```python
from build123d import *

# Parameters (mm, degrees)
SKETCH_4_W           = 84.916455131
SKETCH_4_H           = 80
SKETCH_4_R           = 3
EXTRUDE_1_DEPTH      = 5
EXTRUDE_2_DEPTH      = 3
EXTRUDE_2_DEPTH_BACK = 5
SKETCH_5_R           = 3


with BuildPart() as part:
    # 草图4 → 凸台-拉伸1 (new body)
    with BuildSketch(Plane(origin=(0, 0, 0), x_dir=(1, 0, 0), z_dir=(0, 1, 0))):
        with Locations((-1.967483917, -58.11712094)):
            Rectangle(SKETCH_4_W, SKETCH_4_H)
        with Locations(Location((-36.585071707, -25.636349073, 0), (0, 0, 270))):
            Circle(SKETCH_4_R, mode=Mode.SUBTRACT)
        with Locations(Location((32.601613083, -25.636349073, 0), (0, 0, 270))):
            Circle(SKETCH_4_R, mode=Mode.SUBTRACT)
        with Locations(Location((-36.585071707, -90.861964123, 0), (0, 0, 270))):
            Circle(SKETCH_4_R, mode=Mode.SUBTRACT)
        with Locations(Location((32.601613083, -90.861964123, 0), (0, 0, 270))):
            Circle(SKETCH_4_R, mode=Mode.SUBTRACT)
    extrude(amount=EXTRUDE_1_DEPTH)

    # 草图5 → 凸台-拉伸2 (add, two sides: drawn at the far end of the back side and taken through both)
    with BuildSketch(Plane(origin=(0, 5, 0), x_dir=(1, 0, 0), z_dir=(0, 1, 0)).offset(-EXTRUDE_2_DEPTH_BACK)):
        with Locations(Location((-36.585071707, -25.636349073, 0), (0, 0, 270))):
            Circle(SKETCH_5_R)
        with Locations(Location((32.601613083, -25.636349073, 0), (0, 0, 270))):
            Circle(SKETCH_5_R)
        with Locations(Location((-36.585071707, -90.861964123, 0), (0, 0, 270))):
            Circle(SKETCH_5_R)
        with Locations(Location((32.601613083, -90.861964123, 0), (0, 0, 270))):
            Circle(SKETCH_5_R)
    extrude(amount=EXTRUDE_2_DEPTH + EXTRUDE_2_DEPTH_BACK)


solid = part.part
```
The listing builds one solid part. Answer for the finished solid, in the listing's coordinates (mm). A direction names the side the tool comes from. Coordinates: 2 decimals unless noted, no trailing zeros. Loops run counter-clockwise (first coordinate to the right, second up) from the corner with the lowest first, then second, coordinate; pieces in that order, holes last. Notation, with made-up numbers: (54.25, -22) -> (101.25, -22) arc R14 cw to (101.25, -12) -> close; hole circle Ø6 at (5, 36.25). An arc over 180 degrees is marked (long way). Use one line per item in the form item = value. Start each with the question number.
Item 1: The part is cut by section A-A on z = 80. Determine the outline of the cut face in (x, y).
Item 2: The part is cut by section B-B on y = 7. Determine the outline of the cut face in (x, z).
Item 3: A tool of negligible diameter and unlimited length cuts with its end or side. For faces 5 (the face through (-37, 8, 26)), 6 (the face through (34.63, 6.48, 88.65)), from which of +Z, -Z, +X, -X, +Y, -Y can it reach the whole face along a straight path? Write none if from no direction.
Item 4: The mould has two halves that part along Z. Classify faces 1 (the face through (-3, 2, 18.117)), 2 (the face through (-34.055, 6.479, 27.249)), 3 (the face through (35.13, 6.48, 27.25)), 4 (the face through (33, 8, 26)): released by +Z, released by -Z, zero draft, split by the parting line, or undercut.
Item 5: Consider L1, parallel to Y at x = -10, z = 35; L2, parallel to X at y = 5.75, z = 92; L3, parallel to X at y = 6.25, z = 27.5. Determine where each line is inside the solid, lowest interval first. Write a range as [from, to].
Item 6: The part is cut by section C-C on x = -22. Determine the outline of the cut face in (y, z), then the cut area to 3 significant figures.
Answer key:
q1.outline = (-44.43, 0) -> (40.49, 0) -> (40.49, 5) -> (-44.43, 5) -> close
q2.outline = circle Ø6 at (-36.59, 25.64); circle Ø6 at (-36.59, 90.86); circle Ø6 at (32.6, 25.64); circle Ø6 at (32.6, 90.86)
q3.face_5 = +Z, -Z, +X, -X, +Y
q3.face_6 = +Y
q4.face_1 = released by -Z
q4.face_2 = undercut
q4.face_3 = undercut
q4.face_4 = zero draft
q5.L1 = [0, 5]
q5.L2 = [-39.36, -33.81], [29.83, 35.38]
q5.L3 = [-38.94, -34.23], [30.25, 34.95]
q6.outline = (0, 18.12) -> (5, 18.12) -> (5, 98.12) -> (0, 98.12) -> close
q6.area = 400 mm2
